from build123d import *

# Parameters (mm, degrees)
SKETCH1_R           = 14.307679757
BOSS_EXTRUDE1_DEPTH = 2.5
CUT_EXTRUDE1_DEPTH  = 15
FILLET1_R           = 1
SKETCH6_R           = 1.5
CUT_EXTRUDE2_DEPTH  = 10


with BuildPart() as part:
    # Sketch1 → Boss-Extrude1 (new body)
    with BuildSketch(Plane(origin=(0, 0, 0), x_dir=(1, 0, 0), z_dir=(0, 1, 0))):
        with Locations(Location((0, 0, 0), (0, 0, 270))):
            Circle(SKETCH1_R)
        with BuildLine():
            Line((-2.4, -3.747332385), (2.4, -3.747332385))
            ThreePointArc((2.4, -3.747332385), (0, 4.45), (-2.4, -3.747332385))
        make_face(mode=Mode.SUBTRACT)
    extrude(amount=BOSS_EXTRUDE1_DEPTH)

    # Sketch4 → Cut-Extrude1 (cut)
    with BuildSketch(Plane.XZ):
        with BuildLine():
            Line((-1.2, -4.285148772), (-1.2, -14.257268323))
            ThreePointArc((-1.2, -14.257268323), (0, -14.307679757), (1.2, -14.257268323))
            Line((1.2, -14.257268323), (1.2, -4.285148772))
            ThreePointArc((1.2, -4.285148772), (0, -4.45), (-1.2, -4.285148772))
        make_face()
    extrude(amount=-CUT_EXTRUDE1_DEPTH, mode=Mode.SUBTRACT)

    # Fillet1
    fillet1_edges = [part.edges().sort_by_distance(p)[0] for p in [
        (14.295071343, 2.5, 0.600529207),
        (14.295071343, 0, 0.600529207),
        (1.2, 1.25, -14.257268323),
        (-1.2, 1.25, -14.257268323),
    ]]
    fillet(fillet1_edges, radius=FILLET1_R)

    # Sketch6 → Cut-Extrude2 (cut)
    with BuildSketch(Plane(origin=(0, 2.5, 0), x_dir=(1, 0, 0), z_dir=(0, 1, 0))):
        with Locations(Location((8, 0, 0), (0, 0, 270))):
            Circle(SKETCH6_R)
        with Locations(Location((-8, 0, 0), (0, 0, 270))):
            Circle(SKETCH6_R)
    extrude(amount=-CUT_EXTRUDE2_DEPTH, mode=Mode.SUBTRACT)


solid = part.part
For this review, take the finished solid that the model builds, in its own axes (mm). A direction names the side the tool comes from. Coordinates: 2 decimals unless noted, no trailing zeros. Loops run counter-clockwise (first coordinate to the right, second up) from the corner with the lowest first, then second, coordinate; pieces in that order, holes last. Notation, with made-up numbers: (-2.5, -24.75) - (37.5, -24.75) arc R7 cw to (37.5, -15.75) - close; hole circle Ø10 at (52.5, 23). An arc over 180 degrees is marked (long way). Use a Markdown table: item, result. Add a question column.
Item 1: Insertion check: pin 1 Ø1 at (y, z) = (0.5, -1.5) entering from -X; pin 2 Ø1 at (x, y) = (-9, 0.5) entering from -Z; pin 3 Ø1.2 at (y, z) = (1, -7.5) entering from +X. Each pin has a flat end and moves straight along its axis. Give the tip position at first contact, or say it passes through.
Item 2: Mouldability with a two-part tool opening along X and no side actions: class faces 1 (the face through (0, 2.5, 6)), 2 (the face through (-0.596, 1.246, 14.295)), 3 (the face through (-1.43, 1.27, -13.76)) as pulls with the +X half, pulls with the -X half, needs draft (parallel to the pull), parting line crosses it, or undercut.
Item 3: Tool access review of faces 4 (the face through (4.41, 1.23, -0.59)), 5 (the face through (0, 0, 6)), 6 (the face through (1.2, 1, -9)): name each direction out of +Z, -Z, +X, -X, +Y, -Y from which nothing blocks a thin tool from reaching the whole face with its end or side.
Item 4: For line 1 (X direction, y = 1.4, z = 0); line 2 (X direction, y = 1.9, z = 0); line 3 (Z direction, x = 0, y = 1.1), list the stretches that pass through material, from the lowest coordinate up.
Item 5: We need section A-A (z = 0). Give the boundary of the cut face in (x, y), and give its area (3 significant figures).
Item 6: We need section B-B (x = 0). Give the boundary of the cut face in (y, z).
Results list:
| question | item | result |
|---|---|---|
| 1 | pin 1 | stops at x = -14.25 |
| 1 | pin 2 | stops at z = -11.42 |
| 1 | pin 3 | stops at x = 12.53 |
| 2 | face 1 | needs draft |
| 2 | face 2 | parting line crosses it |
| 2 | face 3 | undercut |
| 3 | face 4 | +Y, -Y |
| 3 | face 5 | +Z, -Z, +X, -X, -Y |
| 3 | face 6 | -Z, +Y, -Y |
| 4 | line 1 | x = -14.31 to -9.5, -6.5 to -4.45, 4.45 to 6.5, 9.5 to 14.31 |
| 4 | line 2 | x = -14.22 to -9.5, -6.5 to -4.45, 4.45 to 6.5, 9.5 to 14.22 |
| 4 | line 3 | z = 3.75 to 14.31 |
| 5 | outline | (-14.31, 1) arc R1 ccw to (-13.31, 0) - (-9.5, 0) - (-9.5, 2.5) - (-13.31, 2.5) arc R1 ccw to (-14.31, 1.5) - close; (-6.5, 0) - (-4.45, 0) - (-4.45, 2.5) - (-6.5, 2.5) - close; (4.45, 0) - (6.5, 0) - (6.5, 2.5) - (4.45, 2.5) - close; (9.5, 0) - (13.31, 0) arc R1 ccw to (14.31, 1) - (14.31, 1.5) arc R1 ccw to (13.31, 2.5) - (9.5, 2.5) - close |
| 5 | area | 33.4 mm^2 |
| 6 | outline | (0, 3.75) - (2.5, 3.75) - (2.5, 13.31) arc R1 ccw to (1.5, 14.31) - (1, 14.31) arc R1 ccw to (0, 13.31) - close |
